```python
from build123d import *

# Parameters (mm, degrees)
SKETCH2_W           = 110
SKETCH2_H           = 20
BOSS_EXTRUDE1_DEPTH = 5
SKETCH3_W           = 85
SKETCH3_H           = 110
BOSS_EXTRUDE2_DEPTH = 3
SKETCH4_R           = 2.3
CUT_EXTRUDE2_DEPTH  = 10
SKETCH5_R           = 1.498794896
CUT_EXTRUDE3_DEPTH  = 10
CUT_EXTRUDE4_DEPTH  = 10


with BuildPart() as part:
    # Sketch2 → Boss-Extrude1 (new body)
    with BuildSketch(Plane(origin=(0, 0, 0), x_dir=(0, 0, -1), z_dir=(1, 0, 0))):
        Rectangle(SKETCH2_W, SKETCH2_H)
    extrude(amount=BOSS_EXTRUDE1_DEPTH)

    # Sketch3 → Boss-Extrude2 (add)
    with BuildSketch(Plane(origin=(0, -10, 0), x_dir=(1, 0, 0), z_dir=(0, 1, 0))):
        with Locations((47.5, 0)):
            Rectangle(SKETCH3_W, SKETCH3_H)
    extrude(amount=BOSS_EXTRUDE2_DEPTH)

    # Sketch4 → Cut-Extrude2 (cut)
    with BuildSketch(Plane(origin=(0, 0, 0), x_dir=(0, 0, -1), z_dir=(1, 0, 0))):
        with Locations(Location((40, 0, 0), (0, 0, 180))):
            Circle(SKETCH4_R)
        with Locations(Location((-40, 0, 0), (0, 0, 180))):
            Circle(SKETCH4_R)
    extrude(amount=CUT_EXTRUDE2_DEPTH, mode=Mode.SUBTRACT)

    # Sketch5 → Cut-Extrude3 (cut)
    with BuildSketch(Plane.XZ.offset(10)):
        with Locations(Location((9, 50.925, 0), (0, 0, 270))):
            Circle(SKETCH5_R)
        with Locations(Location((85.3, 50.925, 0), (0, 0, 270))):
            Circle(SKETCH5_R)
        with Locations(Location((85.3, -50.925, 0), (0, 0, 270))):
            Circle(SKETCH5_R)
        with Locations(Location((9, -50.925, 0), (0, 0, 270))):
            Circle(SKETCH5_R)
    extrude(amount=-CUT_EXTRUDE3_DEPTH, mode=Mode.SUBTRACT)

    # Sketch6 → Cut-Extrude4 (cut)
    with BuildSketch(Plane(origin=(0, -7, 0), x_dir=(1, 0, 0), z_dir=(0, 1, 0))):
        Polygon((80, 35.510778555), (53.397423626, 0), (80, -35.510778555), align=None)
        Polygon((40.903082344, 0.079509445), (13.850723409, -35.089828613), (14.754597533, 35.925976571), align=None)
        Polygon((19.79313121, 45), (47.203523895, 8.410897837), (74.613916581, 45), align=None)
        Polygon((47.203523895, -8.410897837), (74.613916581, -45), (19.79313121, -45), align=None)
    extrude(amount=-CUT_EXTRUDE4_DEPTH, mode=Mode.SUBTRACT)


solid = part.part
```
Verification items for the finished model (mm, model axes). A direction names the side the tool comes from. Round coordinates to 2 decimals unless told otherwise and drop trailing zeros. Order: outer loops, then holes, each group sorted by start corner. A loop starts at its lowest first (then second) coordinate and runs counter-clockwise, first axis right, second up. Notation, with made-up numbers: (81, 10) - (140, 10) arc R16 cw to (140, 19) - close; hole circle Ø5 at (87.5, 39.25). An arc over 180 degrees is marked (long way). Use CSV: the item, a comma, the result in double quotes.
(1) Access from +Z, -Z, +X, -X, +Y, -Y to the whole of each face (thin tool, end or side, straight path). Record for faces 1 (the face through (80, -8, 0)), 2 (the face through (90, -9, 1)).
Entries:
face 1,"+Y, -Y"
face 2,"+Z, -Z, +X, +Y, -Y"
(2) Section check C-C on z = -13. Record the boundary of the cut face in (x, y), and give its area (3 significant figures).
Entries:
outline,"(0, -10) - (14.46, -10) - (14.46, -7) - (5, -7) - (5, 10) - (0, 10) - close; (31.48, -10) - (43.77, -10) - (43.77, -7) - (31.48, -7) - close; (50.64, -10) - (63.14, -10) - (63.14, -7) - (50.64, -7) - close; (80, -10) - (90, -10) - (90, -7) - (80, -7) - close"
area,"233 mm^2"
(3) Gauge pin test, flat ends, axial feed: pin 1 Ø5 at (x, z) = (67.5, -43) entering from -Y; pin 2 Ø5.5 at (y, z) = (0, -40) entering from +X; pin 3 Ø3.5 at (x, z) = (9, 50.925) entering from +Y. Record the tip position at first contact, or that the pin passes through.
Entries:
pin 1,"y = -10"
pin 2,"x = 5"
pin 3,"y = -7"
(4) Thickness scan on probe 1 along Z at (x, y) = (85.3, -8.45); probe 2 along X at (y, z) = (-8, 32); probe 3 along Z at (x, y) = (51, -8.5). Record the ranges inside material, lowest first. Write a range as from..to.
Entries:
probe 1,"-55..-52.42, -49.43..49.43, 52.42..55"
probe 2,"0..13.89, 16.23..29.53, 64.88..77.37, 80..90"
probe 3,"-55..-45, -13.48..13.48, 45..55"
(5) Section check A-A on y = 0. Record the boundary of the cut face in (x, z).
Entries:
outline,"(0, -55) - (5, -55) - (5, -42.3) - (0, -42.3) - close; (0, -37.7) - (5, -37.7) - (5, 37.7) - (0, 37.7) - close; (0, 42.3) - (5, 42.3) - (5, 55) - (0, 55) - close"
(6) Section check B-B on x = 85.3. Record the boundary of the cut face in (y, z), and give its area (3 significant figures).
Entries:
outline,"(-10, -55) - (-7, -55) - (-7, -52.42) - (-10, -52.42) - close; (-10, -49.43) - (-7, -49.43) - (-7, 49.43) - (-10, 49.43) - close; (-10, 52.42) - (-7, 52.42) - (-7, 55) - (-10, 55) - close"
area,"312 mm^2"
(7) Section check D-D on z = 40. Record the boundary of the cut face in (x, y), and give its area (3 significant figures).
Entries:
outline,"(0, -10) - (23.54, -10) - (23.54, -7) - (5, -7) - (5, -2.3) - (0, -2.3) - close; (0, 2.3) - (5, 2.3) - (5, 10) - (0, 10) - close; (70.87, -10) - (90, -10) - (90, -7) - (70.87, -7) - close"
area,"190 mm^2"
(8) Mould release check, pull along Z, two halves, no side actions. Record for faces 3 (the face through (33.31, -8.48, -26.96)), 4 (the face through (47, -7, -1)), 5 (the face through (31.5, -7.5, -55)): released by +Z, released by -Z, zero draft, split by the parting line, or undercut.
Entries:
face 3,"undercut"
face 4,"zero draft"
face 5,"released by -Z"
